from build123d import *

# Parameters (mm, degrees)
F0_R     = 1.4732
F0_W     = 1.74625
F0_H     = 10.15
F0_W_2   = 10.15
F0_H_2   = 1.74625
F1_DEPTH = 1.5875
F2_R     = 4.99999


# Not quite as in the source:
# - a fillet or chamfer is up to 0.001 mm smaller than in the source, because OpenCascade refuses the exact size
# - a length typed as a fraction of an inch, garbled in the dataset ("3 / 203.2 mm" for 3/8 in), is restored


with BuildPart() as f1:
    # F0 (on Right) → F1 (new body)
    with BuildSketch(Plane.YZ):
        Polygon((20, -20), (20, 20), (-20, 20), (-20, -20), (-10, -20), (-10, 10), (10, 10), (10, -20), align=None)
        with Locations((-15, -15)):
            Circle(F0_R, mode=Mode.SUBTRACT)
        with Locations((15, -15)):
            Circle(F0_R, mode=Mode.SUBTRACT)
        with Locations((-15, 0)):
            Rectangle(F0_W, F0_H, mode=Mode.SUBTRACT)
        with Locations((-15, 15)):
            Circle(F0_R, mode=Mode.SUBTRACT)
        with Locations((15, 0)):
            Rectangle(F0_W, F0_H, mode=Mode.SUBTRACT)
        with Locations((0, 15)):
            Rectangle(F0_W_2, F0_H_2, mode=Mode.SUBTRACT)
        with Locations((15, 15)):
            Circle(F0_R, mode=Mode.SUBTRACT)
    extrude(amount=F1_DEPTH)

    # F2 (radius 5 in the source; OpenCascade refuses exactly that, so slightly less here)
    f2_edges = [f1.edges().sort_by_distance(p)[0] for p in [
        (0.79375, -20, 20),
        (0.79375, -20, -20),
        (0.79375, -10, 10),
        (0.79375, -10, -20),
        (0.79375, 10, -20),
        (0.79375, 20, -20),
        (0.79375, 10, 10),
        (0.79375, 20, 20),
    ]]
    fillet(f2_edges, radius=F2_R)


solid = f1.part
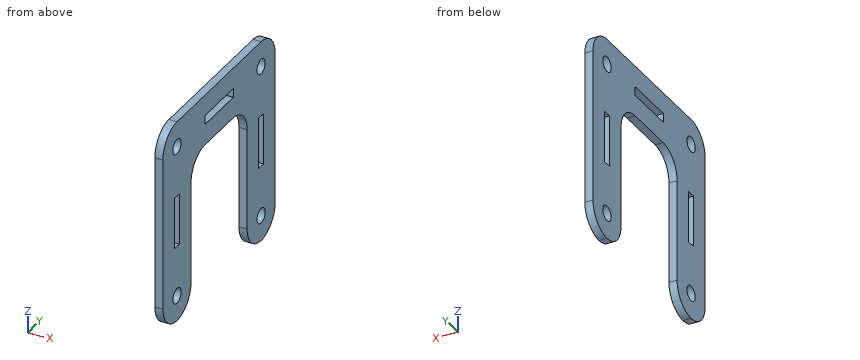
Geometry: final body of the model. Coordinates: model frame, mm. Coordinates: 2 decimals unless noted, no trailing zeros. Order: outer loops, then holes, each group sorted by start corner. A loop starts at its lowest first (then second) coordinate and runs counter-clockwise, first axis right, second up.
1) First-contact query: P1, Ø0.5, axis at x = 1, y = 15.5, coming from the -Z side; P2, Ø4, axis at y = -15, z = 15, coming from the -X side; P3, Ø2, axis at y = 6, z = 8.5, coming from the +X side; P4, Ø0.8, axis at x = 0.5, y = 0, coming from the -Z side. Flat tips, straight axial feed; report the tip coordinate or a pass-through.
Result sheet:
P1: stops at z = -19.99
P2: stops at x = 0
P3: passes through
P4: stops at z = 10
2) Section B-B (x = 1.1). Give the number of separate pieces and of enclosed holes in the cut face, then the cut area to 3 significant figures.
Result sheet:
separate pieces: 1
enclosed holes: 7
area: 898 mm2
3) Section A-A (z = -6). Return loops of the section in (x, y).
Result sheet:
outline: (0, -20) - (1.59, -20) - (1.59, -10) - (0, -10) - close; (0, 10) - (1.59, 10) - (1.59, 20) - (0, 20) - close
4) Ray query, probe 1 along Y at (x, z) = (0.85, -1.5); probe 2 along Z at (x, y) = (1.2, 15) (3 decimals); probe 3 along Z at (x, y) = (0.2, 4). Return the intervals inside material, ascending.
Result sheet:
probe 1: y = -20 to -15.87, -14.13 to -10, 10 to 14.13, 15.87 to 20
probe 2: z = -20 to -16.473, -13.527 to -5.075, 5.075 to 13.527, 16.473 to 20
probe 3: z = 10 to 14.13, 15.87 to 20
5) Section C-C (z = -14). Return loops of the section in (x, y).
Result sheet:
outline: (0, -20) - (1.59, -20) - (1.59, -16.08) - (0, -16.08) - close; (0, -13.92) - (1.59, -13.92) - (1.59, -10) - (0, -10) - close; (0, 10) - (1.59, 10) - (1.59, 13.92) - (0, 13.92) - close; (0, 16.08) - (1.59, 16.08) - (1.59, 20) - (0, 20) - close
6) Section D-D (y = -9). Return loops of the section in (x, z).
Result sheet:
outline: (0, 8) - (1.59, 8) - (1.59, 20) - (0, 20) - close
